```python
from build123d import *

# Parameters (mm, degrees)
SKETCH1_W                                 = 80
SKETCH1_H                                 = 54
BOSS_EXTRUDE2_DEPTH                       = 46.5
FILLET1_R                                 = 2
TIE_START                                 = 17.648406802
TIE_FIGHTER_LAYING_DOWN_BLANK_DEPTH       = 27
TIE_START_2                               = 3.648406802
TIE_FIGHTER_LAYING_DOWN_BLANK_2_OUTLINE_W = 5.5
TIE_FIGHTER_LAYING_DOWN_BLANK_2_OUTLINE_H = 34
TIE_FIGHTER_LAYING_DOWN_BLANK_2_DEPTH     = 14
TIE_START_3                               = 24.148406802
TIE_FIGHTER_LAYING_DOWN_BLANK_3_DEPTH     = 20.5
TIE_START_4                               = 10.648406802
TIE_FIGHTER_LAYING_DOWN_BLANK_4_OUTLINE_R = 2
TIE_FIGHTER_LAYING_DOWN_BLANK_4_DEPTH     = 7
BODY_MOVE_COPY3_ANGLE                     = 90
SKETCH2_W                                 = 7.700906033
SKETCH2_H                                 = 20.169020688
SKETCH2_W_2                               = 7.700906032
CUT_EXTRUDE1_DEPTH                        = 30
SKETCH3_R                                 = 4
CUT_EXTRUDE2_DEPTH                        = 17
SKETCH4_W                                 = 3.700906032
SKETCH4_H                                 = 16.169020688
SKETCH4_W_2                               = 8.420251913
SKETCH4_H_2                               = 21.281008515
SKETCH4_W_3                               = 8.999653324
SKETCH4_W_4                               = 3.700906033
CUT_EXTRUDE3_DEPTH                        = 27
FILLET2_R                                 = 2
SKETCH5_W                                 = 3.700906033
SKETCH5_H                                 = 16.169020688
SKETCH5_W_2                               = 3.700906032
BOSS_EXTRUDE3_DEPTH                       = 2
SKETCH6_R                                 = 4
CUT_EXTRUDE4_DEPTH                        = 11


with BuildPart() as part:
    # Sketch1 → Boss-Extrude2 (new body)
    with BuildSketch(Plane(origin=(0, 0, 0), x_dir=(1, 0, 0), z_dir=(0, 1, 0))):
        with Locations((40, 27)):
            Rectangle(SKETCH1_W, SKETCH1_H)
    extrude(amount=BOSS_EXTRUDE2_DEPTH)

    # Fillet1
    fillet1_edges = [part.edges().sort_by_distance(p)[0] for p in [
        (0, 23.25, -54),
        (80, 23.25, -54),
        (80, 23.25, 0),
        (0, 23.25, 0),
    ]]
    fillet(fillet1_edges, radius=FILLET1_R)


with BuildPart() as body_2:
    # Tie Fighter Laying Down Blank: read off the stored shape, not the designer's step
    # Tie Fighter Laying Down Blank outline → Tie Fighter Laying Down Blank (new body)
    with BuildSketch(Plane(origin=(0, 0, 0), x_dir=(1, 0, 0), z_dir=(0, 1, 0)).offset(TIE_START)):
        with BuildLine():
            Line((-37.161017612, 22.550360254), (-37.161017612, 23.550360254))
            Line((-37.161017612, 23.550360254), (-31.61325597, 23.529243987))
            ThreePointArc((-31.61325597, 23.529243987), (-26.013035095, 20.32886914), (-20.412814219, 23.529243987))
            Line((-20.412814219, 23.529243987), (-14.865052577, 23.550360254))
            Line((-14.865052577, 23.550360254), (-14.865052577, 22.550360254))
            Line((-14.865052577, 22.550360254), (-13.372530837, 22.550360254))
            Line((-13.372530837, 22.550360254), (-13.372530837, 10.033920638))
            Line((-13.372530837, 10.033920638), (-7.872530837, 10.033920638))
            Line((-7.872530837, 10.033920638), (-7.872530837, 44.033920638))
            Line((-7.872530837, 44.033920638), (-13.372530837, 44.033920638))
            Line((-13.372530837, 44.033920638), (-13.372530837, 31.354739987))
            Line((-13.372530837, 31.354739987), (-14.865052577, 31.354739987))
            Line((-14.865052577, 31.354739987), (-14.865052577, 29.979499621))
            Line((-14.865052577, 29.979499621), (-20.327656693, 29.979499621))
            ThreePointArc((-20.327656693, 29.979499621), (-26.013035095, 33.32886914), (-31.698413496, 29.979499621))
            Line((-31.698413496, 29.979499621), (-37.161017612, 29.979499621))
            Line((-37.161017612, 29.979499621), (-37.161017612, 31.354739987))
            Line((-37.161017612, 31.354739987), (-38.653539352, 31.354739987))
            Line((-38.653539352, 31.354739987), (-38.653539352, 44.033920638))
            Line((-38.653539352, 44.033920638), (-44.153539352, 44.033920638))
            Line((-44.153539352, 44.033920638), (-44.153539352, 10.033920638))
            Line((-44.153539352, 10.033920638), (-38.653539352, 10.033920638))
            Line((-38.653539352, 10.033920638), (-38.653539352, 22.550360254))
            Line((-38.653539352, 22.550360254), (-37.161017612, 22.550360254))
        make_face()
    extrude(amount=TIE_FIGHTER_LAYING_DOWN_BLANK_DEPTH)

    # Tie Fighter Laying Down Blank 2 outline → Tie Fighter Laying Down Blank 2 (add)
    with BuildSketch(Plane(origin=(0, 0, 0), x_dir=(1, 0, 0), z_dir=(0, 1, 0)).offset(TIE_START_2)):
        with Locations((-41.403539352, 27.033920638)):
            Rectangle(TIE_FIGHTER_LAYING_DOWN_BLANK_2_OUTLINE_W, TIE_FIGHTER_LAYING_DOWN_BLANK_2_OUTLINE_H)
        with Locations((-10.622530837, 27.033920638)):
            Rectangle(TIE_FIGHTER_LAYING_DOWN_BLANK_2_OUTLINE_W, TIE_FIGHTER_LAYING_DOWN_BLANK_2_OUTLINE_H)
    extrude(amount=TIE_FIGHTER_LAYING_DOWN_BLANK_2_DEPTH)

    # Tie Fighter Laying Down Blank 3 outline → Tie Fighter Laying Down Blank 3 (add)
    with BuildSketch(Plane(origin=(0, 0, 0), x_dir=(1, 0, 0), z_dir=(0, 1, 0)).offset(TIE_START_3)):
        with BuildLine():
            Line((-31.61325597, 23.529243987), (-37.161017612, 23.550360254))
            Line((-37.161017612, 23.550360254), (-37.161017612, 22.550360254))
            Line((-37.161017612, 22.550360254), (-38.653539352, 22.550360254))
            Line((-38.653539352, 22.550360254), (-38.653539352, 20.32886914))
            Line((-38.653539352, 20.32886914), (-26.013035094, 20.32886914))
            ThreePointArc((-26.013035094, 20.32886914), (-29.238127071, 21.18539665), (-31.61325597, 23.529243987))
        make_face()
        with BuildLine():
            ThreePointArc((-20.412814219, 23.529243987), (-22.787943118, 21.18539665), (-26.013035094, 20.32886914))
            Line((-26.013035094, 20.32886914), (-13.372530837, 20.32886914))
            Line((-13.372530837, 20.32886914), (-13.372530837, 22.550360254))
            Line((-13.372530837, 22.550360254), (-14.865052577, 22.550360254))
            Line((-14.865052577, 22.550360254), (-14.865052577, 23.550360254))
            Line((-14.865052577, 23.550360254), (-20.412814219, 23.529243987))
        make_face()
        with BuildLine():
            Line((-38.653539352, 33.32886914), (-38.653539352, 31.354739987))
            Line((-38.653539352, 31.354739987), (-37.161017612, 31.354739987))
            Line((-37.161017612, 31.354739987), (-37.161017612, 29.979499621))
            Line((-37.161017612, 29.979499621), (-31.698413496, 29.979499621))
            ThreePointArc((-31.698413496, 29.979499621), (-29.31234577, 32.429275292), (-26.013035095, 33.32886914))
            Line((-26.013035095, 33.32886914), (-38.653539352, 33.32886914))
        make_face()
        with BuildLine():
            Line((-13.372530837, 33.32886914), (-26.013035095, 33.32886914))
            ThreePointArc((-26.013035095, 33.32886914), (-22.713724419, 32.429275292), (-20.327656693, 29.979499621))
            Line((-20.327656693, 29.979499621), (-14.865052577, 29.979499621))
            Line((-14.865052577, 29.979499621), (-14.865052577, 31.354739987))
            Line((-14.865052577, 31.354739987), (-13.372530837, 31.354739987))
            Line((-13.372530837, 31.354739987), (-13.372530837, 33.32886914))
        make_face()
    extrude(amount=TIE_FIGHTER_LAYING_DOWN_BLANK_3_DEPTH)

    # Tie Fighter Laying Down Blank 4 outline → Tie Fighter Laying Down Blank 4 (add)
    with BuildSketch(Plane(origin=(0, 0, 0), x_dir=(1, 0, 0), z_dir=(0, 1, 0)).offset(TIE_START_4)):
        with Locations((-26.013035095, 26.82886914)):
            Circle(TIE_FIGHTER_LAYING_DOWN_BLANK_4_OUTLINE_R)
    extrude(amount=TIE_FIGHTER_LAYING_DOWN_BLANK_4_DEPTH)


with BuildPart() as body_2_1:
    # Body-Move/Copy2: read off the stored shape, not the designer's step
    # Body-Move/Copy2: moved
    add(body_2.part.moved(Location((0, 1.8515932, 0))))


with BuildPart() as body_2_2:
    # Body-Move/Copy3: moved
    add(body_2_1.part.rotate(Axis((-26.013075057, 0, -27.033920638), (0, 1, 0)), BODY_MOVE_COPY3_ANGLE))


with BuildPart() as body_2_3:
    # Body-Move/Copy4: moved
    add(body_2_2.part.moved(Location((45.307676883, 0, 6.774371597))))


with BuildPart() as body_3:
    # Body-Move/Copy6: read off the stored shape, not the designer's step
    # Body-Move/Copy6: copy of body 2
    add(body_2_3.part.moved(Location((41.4018121, 0, -10.2239757))))


with BuildPart() as body_4:
    # Body-Move_Copy6 2: copy of body 2
    add(body_2_3.part.moved(Location((20.700906, 0, -5.1119878))))


with BuildPart() as body_3_1:
    # Body-Move/Copy7: read off the stored shape, not the designer's step
    # Body-Move/Copy7: moved
    add(body_3.part.moved(Location((0, 0, -2.018363))))


with BuildPart() as body_4_1:
    # Body-Move_Copy7 2: moved
    add(body_4.part.moved(Location((0, 0, -2.018363))))


with BuildPart() as body_2_4:
    # Body-Move_Copy7 3: moved
    add(body_2_3.part.moved(Location((0, 0, -2.018363))))


with BuildPart() as part_1:
    add(part.part)

    # Intersect1: read off the stored shape, not the designer's step
    # Intersect1: cut body 3, body 4, body 2
    add(body_3_1.part, mode=Mode.SUBTRACT)
    add(body_4_1.part, mode=Mode.SUBTRACT)
    add(body_2_4.part, mode=Mode.SUBTRACT)

    # Sketch2 → Cut-Extrude1 (cut)
    with BuildSketch(Plane(origin=(0, 26, 0), x_dir=(1, 0, 0), z_dir=(0, 1, 0))):
        with Locations((29.850106341, 24.833945924)):
            Rectangle(SKETCH2_W, SKETCH2_H)
        with Locations((50.551012373, 29.945933752)):
            Rectangle(SKETCH2_W_2, SKETCH2_H)
    extrude(amount=CUT_EXTRUDE1_DEPTH, mode=Mode.SUBTRACT)

    # Sketch3 → Cut-Extrude2 (cut)
    # profile 1 of 3: a face of its own
    with BuildSketch(Plane.XZ):
        Polygon((38.294601826, -32.918456268), (2, -32.918456268), (2, -11.637447753), (20.995507859, -11.637447753), (20.995507859, -16.74943558), (41.696413892, -16.74943558), (41.696413892, -21.861423408), (78, -21.861423408), (78, -43.142431923), (58.995507859, -43.142431923), (58.995507859, -38.030444096), (38.294601826, -38.030444096), align=None)
        with Locations(Location((60.901465389, -32.501927666, 0), (0, 0, 270))):
            Circle(SKETCH3_R, mode=Mode.SUBTRACT)
        with Locations(Location((40.200559357, -27.389939838, 0), (0, 0, 270))):
            Circle(SKETCH3_R, mode=Mode.SUBTRACT)
        with Locations(Location((19.499653324, -22.277952011, 0), (0, 0, 270))):
            Circle(SKETCH3_R, mode=Mode.SUBTRACT)
    # profile 2 of 3: a face of its own
    with BuildSketch(Plane.XZ):
        Polygon((2.294601826, -42.418456268), (20.995507859, -42.418456268), (20.995507859, -47.530444096), (41.696413892, -47.530444096), (41.696413892, -50.642391961), (41.696413892, -52), (2, -52), (2, -42.418456268), align=None)
    # profile 3 of 3: a face of its own
    with BuildSketch(Plane.XZ):
        Polygon((77.696413892, -12.361423408), (58.995507859, -12.361423408), (58.995507859, -7.24943558), (38.294601826, -7.24943558), (38.294601826, -2), (78, -2), (78, -12.361383446), align=None)
    extrude(amount=-CUT_EXTRUDE2_DEPTH, mode=Mode.SUBTRACT)

    # Sketch4 → Cut-Extrude3 (cut)
    with BuildSketch(Plane.XZ.offset(-17)):
        Polygon((78, -12.361423408), (58.995507859, -12.361423408), (58.995507859, -7.24943558), (38.294601826, -7.24943558), (38.294601826, -2), (58.995507859, -2), (78, -2), align=None)
        Polygon((2, -42.418456268), (20.995507859, -42.418456268), (20.995507859, -47.530444096), (41.696413892, -47.530444096), (41.696413892, -52), (20.995507859, -52), (2, -52), align=None)
        with Locations((50.551012373, -29.945933752)):
            Rectangle(SKETCH4_W, SKETCH4_H)
        with Locations((73.611591346, -32.501927666)):
            Rectangle(SKETCH4_W_2, SKETCH4_H_2)
        with Locations((6.499826662, -22.277952011)):
            Rectangle(SKETCH4_W_3, SKETCH4_H_2)
        with Locations((29.850106341, -24.833945924)):
            Rectangle(SKETCH4_W_4, SKETCH4_H)
    extrude(amount=-CUT_EXTRUDE3_DEPTH, mode=Mode.SUBTRACT)

    # Fillet2
    fillet2_edges = [part_1.edges().sort_by_distance(p)[0] for p in [
        (2, 22, -52),
        (78, 22, -2),
    ]]
    fillet(fillet2_edges, radius=FILLET2_R)

    # Sketch5 → Boss-Extrude3 (add)
    with BuildSketch(Plane(origin=(0, 26, 0), x_dir=(1, 0, 0), z_dir=(0, 1, 0))):
        with Locations((29.850106341, 24.833945924)):
            Rectangle(SKETCH5_W, SKETCH5_H)
        with Locations((50.551012373, 29.945933752)):
            Rectangle(SKETCH5_W_2, SKETCH5_H)
    extrude(amount=-BOSS_EXTRUDE3_DEPTH)

    # Sketch6 → Cut-Extrude4 (cut)
    with BuildSketch(Plane.XZ):
        with Locations(Location((19.499653324, -22.277952011, 0), (0, 0, 270))):
            Circle(SKETCH6_R)
        with Locations(Location((40.200559357, -27.389939838, 0), (0, 0, 270))):
            Circle(SKETCH6_R)
        with Locations(Location((60.901465389, -32.501927666, 0), (0, 0, 270))):
            Circle(SKETCH6_R)
    extrude(amount=-CUT_EXTRUDE4_DEPTH, mode=Mode.SUBTRACT)


solid = part_1.part
```
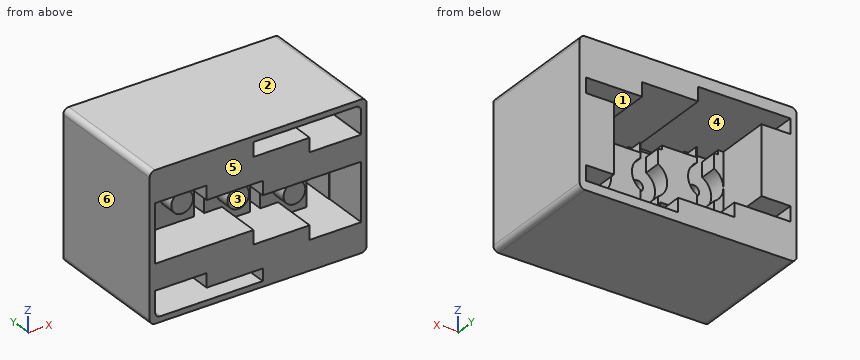
CAD build for the part. Positions are in the model's coordinates, mm. Face numbers are marked on the shaded views. A direction names the side the tool comes from. Coordinates: 2 decimals unless noted, no trailing zeros. Write each loop counter-clockwise with the first axis right and the second up, starting at its lowest first coordinate (ties: lowest second). Pieces come first, ordered by that corner, then holes.
(1) Cut at B-B, the plane z = -41.5. List the corners of the cut face in (x, y).
(2) Drill centre lines: probe 1 along X at (y, z) = (42, -4.5); probe 2 along Z at (x, y) = (26.5, 18); probe 3 along X at (y, z) = (22, -40). Where is each one in solid material? Low to high.
(3) Cut at A-A, the plane y = 7. Count the separate pieces of the cut face and the enclosed holes in it, and give its area (3 significant figures).
(4) Flat gauge pins, fed straight in: pin 1 (1.7 mm diameter, centred on x = 14, z = -26.5, fed in from +Y); pin 2 (3 mm diameter, centred on x = 60.9, z = -32.5, fed in from -Y). Where does each tip first touch, or does it go through?
(5) Cut at D-D, the plane z = -13.5. List the corners of the cut face in (x, y).
(6) 3-axis set-ups, long thin cutter, end or side, ignore diameter. For the marked faces 1, 2 and 3: which of +Z, -Z, +X, -X, +Y, -Y reach the whole face in a straight line?
(7) Two-plate mould, pull along X, no slides. Class the marked faces 4, 5 and 6: +X half, -X half, draft (parallel to the pull), parting line (faces both ways), or undercut.
Geometry says:
1. outline: (0, 0) - (59, 0) - (59, 17) - (69.4, 17) - (69.4, 44) - (77.82, 44) - (77.82, 17) - (78, 17) - (78, 0) - (80, 0) - (80, 46.5) - (67.4, 46.5) - (67.4, 26) - (64.19, 26) - (64.19, 19.5) - (57.75, 19.5) - (57.75, 26) - (57, 26) - (57, 5.5) - (23, 5.5) - (23, 46.5) - (0, 46.5) - close
2. probe 1: x = 0 to 2.29, 36.29 to 38.29, 78 to 80
2. probe 2: z = -54 to -52, -47.53 to -45.53, -34.92 to -14.75, -4.14 to 0
2. probe 3: x = 0 to 2.29, 44.48 to 57.75, 64.19 to 69.4, 77.82 to 80
3. separate pieces: 1
3. enclosed holes: 5
3. area: 1,200 mm2
4. pin 1: stops at y = 26
4. pin 2: stops at y = 11
5. outline: (0, 0) - (2, 0) - (2, 44) - (11, 44) - (11, 17) - (21, 17) - (21, 0) - (80, 0) - (80, 46.5) - (57, 46.5) - (57, 5.5) - (23, 5.5) - (23, 26) - (22.79, 26) - (22.79, 19.5) - (16.35, 19.5) - (16.35, 26) - (13, 26) - (13, 46.5) - (0, 46.5) - close
6. face 1: +Y
6. face 2: +Z, +X, -X, +Y, -Y
6. face 3: -Y
7. face 4: undercut
7. face 5: draft
7. face 6: -X half
